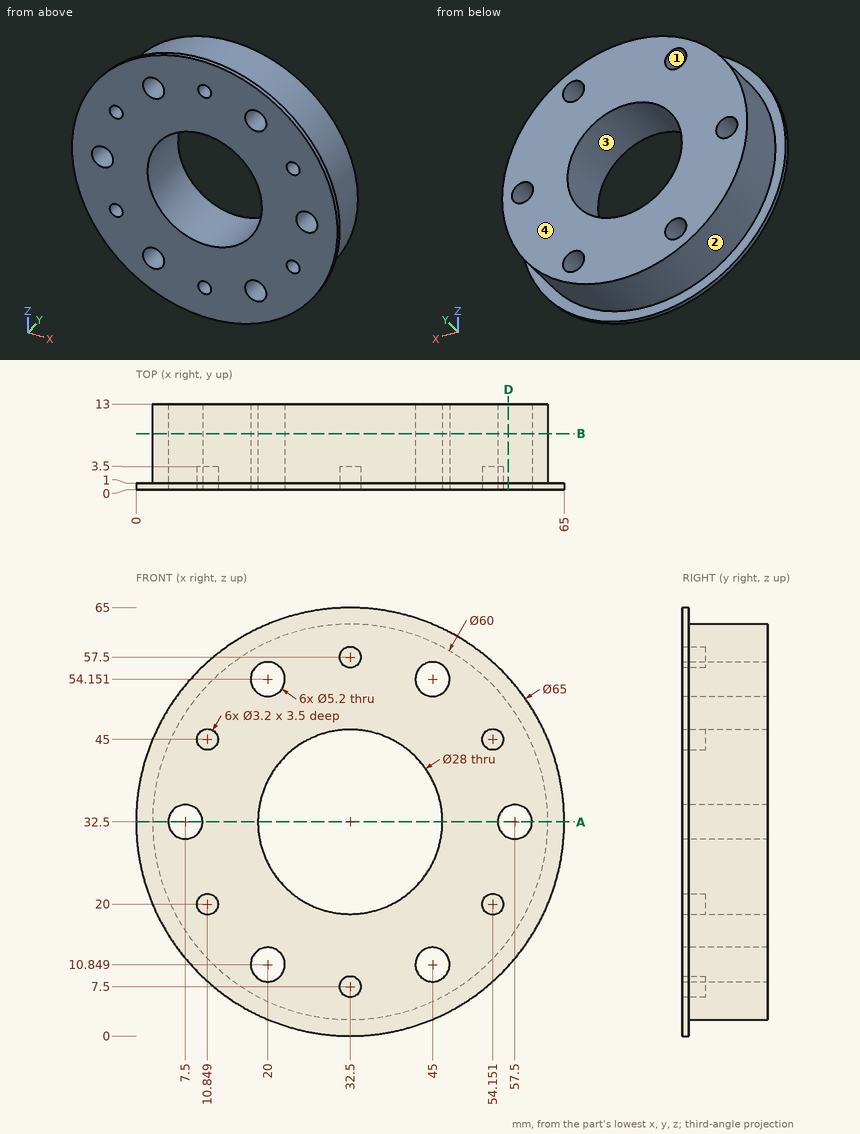
Drawing for the job (mm, zero at the part's lowest x, y, z). Coordinates: 2 decimals unless noted, no trailing zeros. Loops run counter-clockwise (first coordinate to the right, second up) from the corner with the lowest first, then second, coordinate; pieces in that order, holes last. Notation, with made-up numbers: (36.5, -9.75) - (55.5, -9.75) arc R20 ccw to (55.5, -1.75) - close; hole circle Ø1 at (41.25, -13). An arc over 180 degrees is marked (long way). Return JSON: item names as keys, results as strings.
1. Probe L1, parallel to X at y = 3.25, z = 32.5; L2, parallel to X at y = 3, z = 55 (1 decimal); L3, parallel to Z at x = 43.5, y = 9.5 (1 decimal). List the from-to ranges inside material, lowest first. Write a range as from..to.
Result:
{"L1": "x = 2.5..4.9, 10.1..18.5, 46.5..54.9, 60.1..62.5", "L2": "x = 12.7..17.5, 22.5..42.5, 47.5..52.3", "L3": "z = 4.6..8.7, 13..23.8, 41.2..52, 56.3..60.4"}
2. Band-saw the part on B-B (y = 8.5). Give the cut face in (x, z).
Result:
{"outline": "circle Ø60 at (32.5, 32.5); hole circle Ø5.2 at (7.5, 32.5); hole circle Ø5.2 at (20, 10.85); hole circle Ø5.2 at (20, 54.15); hole circle Ø28 at (32.5, 32.5); hole circle Ø5.2 at (45, 10.85); hole circle Ø5.2 at (45, 54.15); hole circle Ø5.2 at (57.5, 32.5)"}
3. Mould opens along X. For the marked faces 1, 2, 3 and 4 say: released by +X, released by -X, zero draft, split by the parting line, or undercut.
Result:
{"face 1": "undercut", "face 2": "split by the parting line", "face 3": "undercut", "face 4": "zero draft"}
4. Band-saw the part on D-D (x = 56.5). Give the cut face in (y, z) (1 decimal).
Result:
{"outline": "(0, 10.6) - (1, 10.6) - (1, 14.5) - (13, 14.5) - (13, 30.1) - (0, 30.1) - close; (0, 34.9) - (13, 34.9) - (13, 50.5) - (1, 50.5) - (1, 54.4) - (0, 54.4) - close"}
5. Drop flat-ended pins along their axis: pin 1 (1 mm diameter, centred on x = 11.5, z = 44.5, fed in from -Y); pin 2 (6 mm diameter, centred on x = 7.5, z = 32.5, fed in from -Y); pin 3 (4 mm diameter, centred on y = 7.5, z = 55, fed in from +X); pin 4 (4 mm diameter, centred on x = 17.5, y = 5, fed in from +Z). Give the stop position or say it passes through.
Result:
{"pin 1": "stops at y = 3.5", "pin 2": "stops at y = 0", "pin 3": "stops at x = 54.4", "pin 4": "stops at z = 59.54"}
6. Band-saw the part on A-A (z = 32.5). Give the cut face in (x, y).
Result:
{"outline": "(0, 0) - (4.9, 0) - (4.9, 13) - (2.5, 13) - (2.5, 1) - (0, 1) - close; (10.1, 0) - (18.5, 0) - (18.5, 13) - (10.1, 13) - close; (46.5, 0) - (54.9, 0) - (54.9, 13) - (46.5, 13) - close; (60.1, 0) - (65, 0) - (65, 1) - (62.5, 1) - (62.5, 13) - (60.1, 13) - close"}
